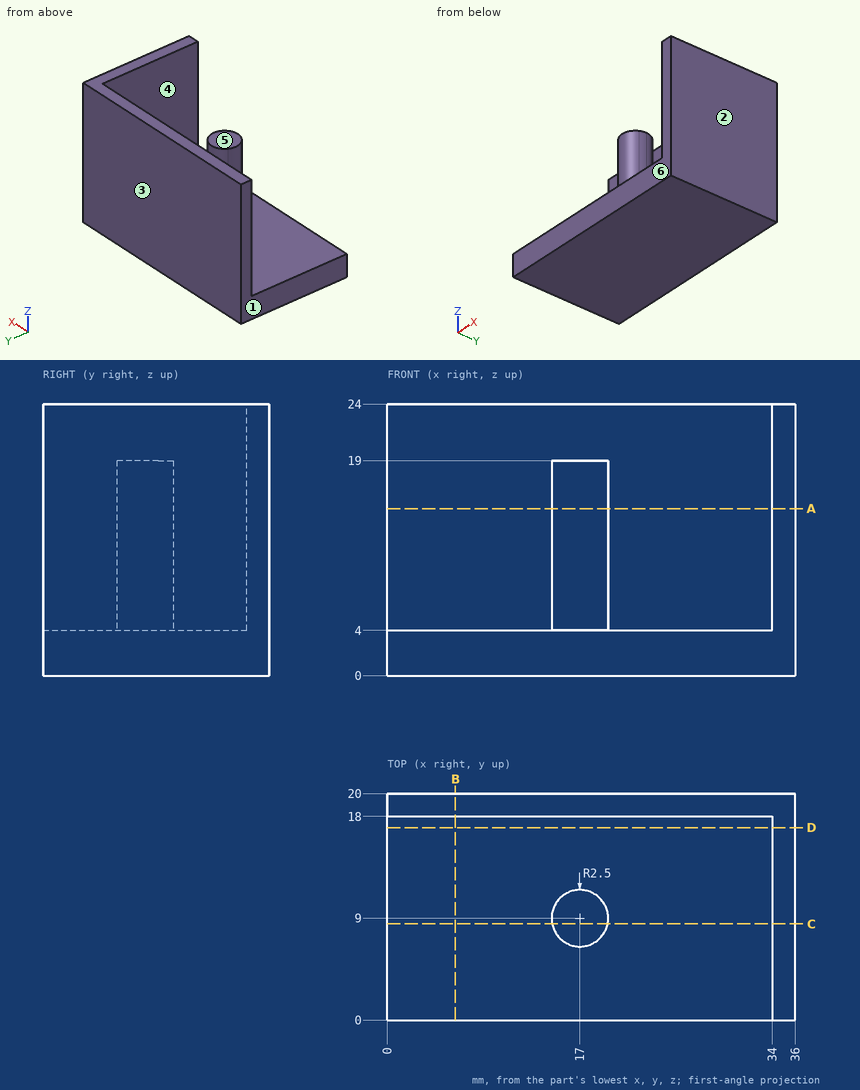
Print and shaded views of the part. All mm, measured from the part's lowest x, y and z. A direction names the side the tool comes from. Coordinates: 2 decimals unless noted, no trailing zeros. Loops run counter-clockwise (first coordinate to the right, second up) from the corner with the lowest first, then second, coordinate; pieces in that order, holes last. Notation, with made-up numbers: (-21.75, 23.25) -> (35.25, 23.25) arc R19 cw to (35.25, 49.25) -> close; hole circle Ø4 at (56.25, 71.5). An arc over 180 degrees is marked (long way). Use a Markdown table: item, result. Add a question column.
Item 1: Band-saw the part on B-B on x = 6. Write the cut outline in (y, z).
Item 2: Band-saw the part on C-C on y = 8.5. Write the cut outline in (x, z), plus the area to 3 significant figures.
Item 3: Band-saw the part on A-A on z = 14.75. Write the cut outline in (x, y).
Item 4: Which spindle directions (+Z, -Z, +X, -X, +Y, -Y) get a long thin tool onto all of the face, cutting with end or side? Do the marked faces 5 and 6. Say none if no direction does.
Item 5: Flat gauge pins, fed straight in: P1, Ø5.5, axis at y = 7, z = 18.5, coming from the -X side; P2, Ø1.5, axis at x = 32.5, y = 3, coming from the +Z side; P3, Ø1.5, axis at y = 3.5, z = 9, coming from the -X side. Where does each tip first touch, or does it go through?
Item 6: Band-saw the part on D-D on y = 17. Write the cut outline in (x, z), plus the area to 3 significant figures.
Item 7: Pull direction X, two halves, no side cores. Call the marked faces 1, 2, 3 and 4: +X half, -X half, draft (parallel to the pull), parting line (faces both ways), or undercut.
Item 8: Probe probe 1 along X at (y, z) = (9, 17.75); probe 2 along Z at (x, y) = (6, 9.5); probe 3 along Y at (x, z) = (11.5, 19.5). List the from-to ranges inside material, lowest first.
Geometry says:
| question | item | result |
|---|---|---|
| 1 | outline | (0, 0) -> (20, 0) -> (20, 24) -> (18, 24) -> (18, 4) -> (0, 4) -> close |
| 2 | outline | (0, 0) -> (36, 0) -> (36, 24) -> (34, 24) -> (34, 4) -> (19.45, 4) -> (19.45, 19) -> (14.55, 19) -> (14.55, 4) -> (0, 4) -> close |
| 2 | area | 257 mm² |
| 3 | outline | (0, 18) -> (34, 18) -> (34, 0) -> (36, 0) -> (36, 20) -> (0, 20) -> close; (19.21, 7.83) arc R2.5 ccw to (19.5, 9) arc R2.5 ccw to (19.21, 10.17) arc R2.5 ccw (long way) to start |
| 4 | face 5 | +Z, -X, -Y |
| 4 | face 6 | +Z, -Z, +X, -X, -Y |
| 5 | P1 | x = 14.5 |
| 5 | P2 | z = 4 |
| 5 | P3 | x = 34 |
| 6 | outline | (0, 0) -> (36, 0) -> (36, 24) -> (34, 24) -> (34, 4) -> (0, 4) -> close |
| 6 | area | 184 mm² |
| 7 | face 1 | -X half |
| 7 | face 2 | +X half |
| 7 | face 3 | draft |
| 7 | face 4 | undercut |
| 8 | probe 1 | 14.5 to 19.5, 34 to 36 |
| 8 | probe 2 | 0 to 4 |
| 8 | probe 3 | 18 to 20 |
